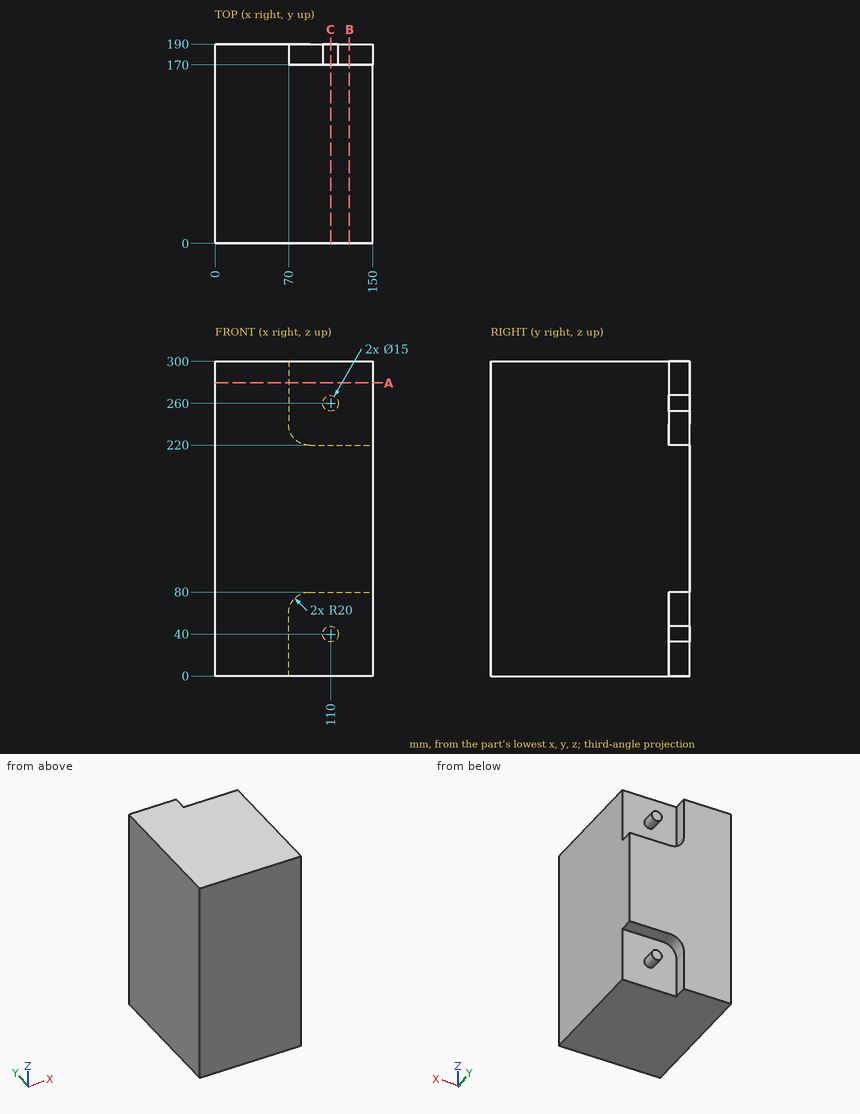
For this review, use the dimensioned drawing (mm, ordinates from the lowest corner) and the shaded views. Round coordinates to 2 decimals unless told otherwise and drop trailing zeros. Loops run counter-clockwise (first coordinate to the right, second up) from the corner with the lowest first, then second, coordinate; pieces in that order, holes last. Notation, with made-up numbers: M 87,32.25 L 115,32.25 A13 ccw 115,36.25 Z; hole C -7.75,-20 d6. An arc over 180 degrees is marked long. Answer as CSV lines item,"result".
1. To check wall thickness, follow L1, parallel to Y at x = 84, z = 48. State the ranges of the line that lie inside material, in increasing order. Write a range as [from, to].
Outcome:
L1,"y = [0, 170]"
2. We need section A-A (z = 279.5). Give the boundary of the cut face in (x, y).
Outcome:
outline,"M 0,0 L 150,0 L 150,170 L 70,170 L 70,190 L 0,190 Z"
3. We need section C-C (x = 110). Give the boundary of the cut face in (y, z).
Outcome:
outline,"M 0,0 L 170,0 L 170,32.5 L 190,32.5 L 190,47.5 L 170,47.5 L 170,80 L 190,80 L 190,220 L 170,220 L 170,252.5 L 190,252.5 L 190,267.5 L 170,267.5 L 170,300 L 0,300 Z"
4. Insertion check: pin 1 Ø8 at (x, z) = (72, 51) entering from -Y; pin 2 Ø16 at (x, y) = (122, 184) entering from -Z; pin 3 Ø10 at (y, z) = (182, 19.5) entering from +X; pin 4 Ø6 at (x, y) = (105.5, 180) entering from +Z. Each pin has a flat end and moves straight along its axis. Give the tip position at first contact, or say it passes through.
Outcome:
pin 1,"stops at y = 0"
pin 2,"stops at z = 33.66"
pin 3,"stops at x = 70"
pin 4,"stops at z = 267.35"
5. We need section B-B (x = 128). Give the boundary of the cut face in (y, z).
Outcome:
outline,"M 0,0 L 170,0 L 170,80 L 190,80 L 190,220 L 170,220 L 170,300 L 0,300 Z"
